Geometry check sheet. Reference: the model listing, model coordinates, mm. A direction names the side the tool comes from. Coordinates: 2 decimals unless noted, no trailing zeros. Write each loop counter-clockwise with the first axis right and the second up, starting at its lowest first coordinate (ties: lowest second). Pieces come first, ordered by that corner, then holes. Notation, with made-up numbers: (54, -39) -> (83, -39) arc R13 ccw to (83, -23) -> close; hole circle Ø4 at (76, 15). An arc over 180 degrees is marked (long way). Answer in a Markdown table with one row per item. Add a question column.
1. Set-up check for faces 4 (the cylindrical face through (-32, 2.01, -23.43)), 5 (the flat face through (30, 0.5, 20)), 6 (the cylindrical face through (31.57, 2.01, -23.15)), 7 (the flat face through (-33.5, 2, 0)), 8 (the cylindrical face through (12.989, 4.335, 25.918)): record each of +Z, -Z, +X, -X, +Y, -Y from which the full face is reachable in a straight line by a thin tool's end or side.
2. Mould release check, pull along Z, two halves, no side actions. Record for faces 1 (the cylindrical face through (-7.7, 4.43, 26.4)), 2 (the flat face through (35.5, 1, -5)), 3 (the flat face through (-33, 0.5, -24)): pulls with the +Z half, pulls with the -Z half, needs draft (parallel to the pull), parting line crosses it, or undercut.
3. Scan lines: L1, parallel to Z at x = -33.2, y = 0.1; L2, parallel to Z at x = -28.5, y = 2; L3, parallel to Z at x = -33.2, y = 0.6. Record each from-to range of solid material in increasing order. Write a range as from..to.
4. Cross-section at B-B on z = -15. Record the cut outline in (x, y).
5. Depth check by flat-ended pin: P1, Ø15, axis at x = -10.5, z = -1, coming from the -Y side; P2, Ø2, axis at x = 30, z = 19, coming from the +Y side; P3, Ø4, axis at x = -33, z = -25, coming from the +Y side (3 decimals); P4, Ø0.9, axis at x = 32.5, z = -24.7, coming from the -Y side. Enter the tip coordinate at first touch or a pass-through.
6. Cross-section at A-A on x = 8.5. Record the cut outline in (y, z).
```python
from build123d import *

# Parameters (mm, degrees)
SKETCH1_W                         = 71
SKETCH1_H                         = 54
BOSS_EXTRUDE1_DEPTH               = 5
M1_4X0_3_TAPPED_HOLE1_D           = 1.1
M1_4X0_3_TAPPED_HOLE1_CSINK_D     = 1.45
M1_4X0_3_TAPPED_HOLE1_CSINK_ANGLE = 90
CUT_EXTRUDE1_DEPTH                = 4
SKETCH5_R                         = 6
SKETCH5_R_2                       = 5
SKETCH5_R_3                       = 5.5
CUT_EXTRUDE2_DEPTH                = 4
FILLET1_R                         = 2
FILLET2_R                         = 2
SKETCH6_R                         = 1
CUT_EXTRUDE3_DEPTH                = 0.5


with BuildPart() as part:
    # Sketch1 → Boss-Extrude1 (new body)
    with BuildSketch(Plane(origin=(0, 0, 0), x_dir=(1, 0, 0), z_dir=(0, 1, 0))):
        Rectangle(SKETCH1_W, SKETCH1_H)
    extrude(amount=BOSS_EXTRUDE1_DEPTH)

    # M1.4x0.3 Tapped Hole1 (through all)
    with Locations(Plane(origin=(0, 5, 0), x_dir=(1, 0, 0), z_dir=(0, 1, 0))):
        with Locations((-33.2, 24.7), (32.5, 24.7), (-33.2, -23), (29.4, -19.4)):
            CounterSinkHole(M1_4X0_3_TAPPED_HOLE1_D / 2, M1_4X0_3_TAPPED_HOLE1_CSINK_D / 2, counter_sink_angle=M1_4X0_3_TAPPED_HOLE1_CSINK_ANGLE)

    # Sketch4 → Cut-Extrude1 (cut)
    with BuildSketch(Plane.XZ):
        with BuildLine():
            Line((-7.748076809, 19), (-33.5, 19))
            Line((-33.5, 19), (-33.5, -20))
            Line((-33.5, -20), (-6.5, -20))
            ThreePointArc((-6.5, -20), (33.487208249, 0.799639875), (-7.748076809, 19))
        make_face()
    extrude(amount=-CUT_EXTRUDE1_DEPTH, mode=Mode.SUBTRACT)

    # Sketch5 → Cut-Extrude2 (cut)
    with BuildSketch(Plane(origin=(0, 5, 0), x_dir=(1, 0, 0), z_dir=(0, 1, 0))):
        with Locations((-35.5, -27)):
            Circle(SKETCH5_R)
        with Locations((-35.5, 27)):
            Circle(SKETCH5_R_2)
        with Locations((35.5, 27)):
            Circle(SKETCH5_R_3)
        with BuildLine():
            Line((34.5, -1), (35.5, -1))
            Line((35.5, -1), (35.5, -27))
            Line((35.5, -27), (13.5, -27))
            Line((13.5, -27), (13.5, -26))
            ThreePointArc((13.5, -26), (28.644692027, -17.401541303), (34.5, -1))
        make_face()
    extrude(amount=-CUT_EXTRUDE2_DEPTH, mode=Mode.SUBTRACT)

    # Fillet1
    fillet1_edges = [part.edges().sort_by_distance(p)[0] for p in [
        (35.5, 0.5, 27),
        (-35.5, 0.5, 27),
        (-35.5, 0.5, -27),
        (35.5, 0.5, -27),
    ]]
    fillet(fillet1_edges, radius=FILLET1_R)

    # Fillet2
    fillet2_edges = [part.edges().sort_by_distance(p)[0] for p in [
        (35.5, 5, -10.25),
        (-0.25, 5, -27),
        (-35.5, 5, -0.5),
        (-8, 5, 27),
        (28.644692027, 5, 17.401541303),
        (13.5, 5, 26.5),
        (35, 5, 1),
        (31.610912703, 5, -23.110912703),
        (-31.964466094, 5, -23.464466094),
        (-31.257359313, 5, 22.757359313),
    ]]
    fillet(fillet2_edges, radius=FILLET2_R)

    # Sketch6 → Cut-Extrude3 (cut)
    with BuildSketch(Plane(origin=(0, 1, 0), x_dir=(1, 0, 0), z_dir=(0, 1, 0))):
        with Locations((-33.2, 24.7)):
            Circle(SKETCH6_R)
        with Locations((32.5, 24.7)):
            Circle(SKETCH6_R)
        with Locations((29.4, -19.4)):
            Circle(SKETCH6_R)
        with Locations((-33.2, -23)):
            Circle(SKETCH6_R)
    extrude(amount=-CUT_EXTRUDE3_DEPTH, mode=Mode.SUBTRACT)


solid = part.part
```
Results found:
| question | item | result |
|---|---|---|
| 1 | face 4 | -Z, -X, +Y |
| 1 | face 5 | +Y |
| 1 | face 6 | -Z, +X, +Y |
| 1 | face 7 | -Y |
| 1 | face 8 | +Z, +X, +Y |
| 2 | face 1 | pulls with the +Z half |
| 2 | face 2 | needs draft |
| 2 | face 3 | undercut |
| 3 | L1 | z = -27..-25.25, -24.15..-20, 19..22.45, 23.55..27 |
| 3 | L2 | z = -27..-20, 19..27 |
| 3 | L3 | z = -27..-25.7, -23.7..-20, 19..22, 24..27 |
| 4 | outline | (-35.5, 0) -> (-33.5, 0) -> (-33.5, 4) -> (28.5, 4) -> (28.5, 0) -> (35.5, 0) -> (35.5, 3) arc R2 ccw to (33.5, 5) -> (-33.5, 5) arc R2 ccw to (-35.5, 3) -> close |
| 5 | P1 | stops at y = 4 |
| 5 | P2 | stops at y = 1 |
| 5 | P3 | stops at y = 3.875 |
| 5 | P4 | passes through |
| 6 | outline | (0, -27) -> (3, -27) arc R2 ccw to (5, -25) -> (5, 25) arc R2 ccw to (3, 27) -> (0, 27) -> (0, 25) -> (4, 25) -> (4, -25) -> (0, -25) -> close |
